Geometry: final body of the model. Coordinates: model frame, mm. A direction names the side the tool comes from. Give positions to 0.01 mm unless a question says otherwise; leave off trailing zeros. Write each loop counter-clockwise with the first axis right and the second up, starting at its lowest first coordinate (ties: lowest second). Pieces come first, ordered by that corner, then holes.
Q1. Cut plane D-D on y = 31.5. Return the cut outline in (x, z), plus the area to 3 significant figures.
Q2. Cut plane C-C on x = -35.5. Return the cut outline in (y, z), plus the area to 3 significant figures.
Q3. Draft query along Z for faces 1 (the face through (-40.5, 26, 23)), 2 (the face through (-32, 8, 19)), 3 (the face through (-59, -3, 12)). Return one class per face: pulls with the +Z half, pulls with the -Z half, needs draft (parallel to the pull), parting line crosses it, or undercut.
Q4. Line query: L1, parallel to Z at x = -50, y = 10; L2, parallel to Y at x = -16.5, z = 25.75; L3, parallel to X at y = 12, z = 20. Output: solid intervals per line, ascending.
Q5. Cut plane A-A on y = 11.5. Return the cut outline in (x, z), plus the area to 3 significant figures.
Q6. Pin query (flat end, axial travel): pin 1 (5 mm diameter, centred on x = -50, y = 32, fed in from +Z); pin 2 (5 mm diameter, centred on x = -56.5, y = 24.5, fed in from -Z); pin 3 (2 mm diameter, centred on x = -51, y = 24.5, fed in from -Z). Return the tip coordinate at first contact, or that it passes through.
Q7. Cut plane B-B on x = -44. Return the cut outline in (y, z), plus the area to 3 significant figures.
Q8. Reachability of faces 4 (the face through (-54, 26, 16)), 5 (the face through (-30, 0, 15)), 6 (the face through (-38, 14, 18)), 7 (the face through (-40, 26, 24)) from +Z, -Z, +X, -X, +Y, -Y: full face, straight path, thin tool, end or side. Return the list, or none.
```python
from build123d import *

# Parameters (mm, degrees)
ESQUISSE5_W             = 60
ESQUISSE5_H             = 30
BOSS_EXTRU_2_DEPTH      = 15
ESQUISSE6_R             = 5
BOSS_EXTRU_3_DEPTH      = 6
BOSS_EXTRU_4_DEPTH      = 23
ESQUISSE8_W             = 50
ESQUISSE8_H             = 3
ENL_V_MAT_EXTRU_1_DEPTH = 7
ESQUISSE9_W             = 7
ESQUISSE9_H             = 7
ENL_V_MAT_EXTRU_2_DEPTH = 7


with BuildPart() as part:
    # Esquisse5 → Boss.-Extru.2 (new body)
    with BuildSketch(Plane(origin=(0, 0, 0), x_dir=(1, 0, 0), z_dir=(0, 1, 0))):
        with Locations((-30, -15)):
            Rectangle(ESQUISSE5_W, ESQUISSE5_H)
    extrude(amount=BOSS_EXTRU_2_DEPTH)

    # Esquisse6 → Boss.-Extru.3 (add)
    with BuildSketch(Plane.XZ):
        with Locations((-55, 15)):
            Circle(ESQUISSE6_R)
        with Locations((-15, 15)):
            Circle(ESQUISSE6_R)
    extrude(amount=BOSS_EXTRU_3_DEPTH)

    # Esquisse7 → Boss.-Extru.4 (add)
    with BuildSketch(Plane(origin=(0, 15, 0), x_dir=(1, 0, 0), z_dir=(0, 1, 0))):
        Polygon((-60, -15), (-54, -15), (-54, -18), (-57, -18), (-57, -21), (-28, -21), (-28, -24), (-60, -24), align=None)
    extrude(amount=BOSS_EXTRU_4_DEPTH)

    # Esquisse8 → Enlèv. mat.-Extru.1 (cut)
    with BuildSketch(Plane(origin=(0, 15, 0), x_dir=(1, 0, 0), z_dir=(0, 1, 0))):
        with Locations((-32, -19.5)):
            Rectangle(ESQUISSE8_W, ESQUISSE8_H)
    extrude(amount=-ENL_V_MAT_EXTRU_1_DEPTH, mode=Mode.SUBTRACT)

    # Esquisse9 → Enlèv. mat.-Extru.2 (cut)
    with BuildSketch(Plane.XY.offset(24)):
        with Locations((-44, 26.5)):
            Rectangle(ESQUISSE9_W, ESQUISSE9_H)
    extrude(amount=-ENL_V_MAT_EXTRU_2_DEPTH, mode=Mode.SUBTRACT)


solid = part.part
```
Data:
1. outline: (-60, 15) - (-54, 15) - (-54, 18) - (-57, 18) - (-57, 21) - (-28, 21) - (-28, 24) - (-60, 24) - close
1. area: 123 mm2
2. outline: (0, 0) - (15, 0) - (15, 18) - (8, 18) - (8, 21) - (38, 21) - (38, 24) - (15, 24) - (15, 30) - (0, 30) - close
2. area: 498 mm2
3. face 1: needs draft
3. face 2: undercut
3. face 3: parting line crosses it
4. L1: z = 0 to 18, 21 to 30
4. L2: y = 0 to 15
4. L3: x = -60 to -57, -7 to 0
5. outline: (-60, 0) - (0, 0) - (0, 30) - (-60, 30) - close; hole (-57, 18) - (-7, 18) - (-7, 21) - (-57, 21) - close
5. area: 1,650 mm2
6. pin 1: stops at z = 24
6. pin 2: stops at z = 15
6. pin 3: stops at z = 21
7. outline: (0, 0) - (15, 0) - (15, 18) - (8, 18) - (8, 21) - (23, 21) - (23, 24) - (15, 24) - (15, 30) - (0, 30) - close; (30, 21) - (38, 21) - (38, 24) - (30, 24) - close
7. area: 477 mm2
8. face 4: -Z, +X, +Y
8. face 5: -Y
8. face 6: +Y
8. face 7: +Z, +X, -X, +Y
